```python
from build123d import *

# Parameters (mm, degrees)
ESQUISSE1_R        = 55
ESQUISSE1_R_2      = 1.227
ESQUISSE1_R_3      = 5
BOSS_EXTRU_1_DEPTH = 5
CONG_1_R           = 3
CHANFREIN1_SIZE    = 1


with BuildPart() as part:
    # Esquisse1 → Boss.-Extru.1 (new body)
    with BuildSketch(Plane.XY):
        Circle(ESQUISSE1_R)
        with Locations((-41.13620668, 23.75)):
            Circle(ESQUISSE1_R_2, mode=Mode.SUBTRACT)
        with Locations((-41.13620668, -23.75)):
            Circle(ESQUISSE1_R_2, mode=Mode.SUBTRACT)
        with Locations((0, -47.5)):
            Circle(ESQUISSE1_R_2, mode=Mode.SUBTRACT)
        with Locations((41.13620668, -23.75)):
            Circle(ESQUISSE1_R_2, mode=Mode.SUBTRACT)
        with Locations((41.13620668, 23.75)):
            Circle(ESQUISSE1_R_2, mode=Mode.SUBTRACT)
        with Locations((0, 47.5)):
            Circle(ESQUISSE1_R_2, mode=Mode.SUBTRACT)
        Circle(ESQUISSE1_R_3, mode=Mode.SUBTRACT)
        with BuildLine():
            ThreePointArc((36.043450899, -17.345594464), (34.641016151, 20), (3, 39.88734135))
            Line((3, 39.88734135), (3, 9.539392014))
            ThreePointArc((3, 9.539392014), (8.660254038, 5), (9.761355821, -2.171619796))
            Line((9.761355821, -2.171619796), (36.043450899, -17.345594464))
        make_face(mode=Mode.SUBTRACT)
        with BuildLine():
            ThreePointArc((-33.043450899, -22.541746887), (0, -40), (33.043450899, -22.541746887))
            Line((33.043450899, -22.541746887), (6.761355821, -7.367772218))
            ThreePointArc((6.761355821, -7.367772218), (0, -10), (-6.761355821, -7.367772218))
            Line((-6.761355821, -7.367772218), (-33.043450899, -22.541746887))
        make_face(mode=Mode.SUBTRACT)
        with BuildLine():
            Line((-3, 9.539392014), (-3, 39.88734135))
            ThreePointArc((-3, 39.88734135), (-34.641016151, 20), (-36.043450899, -17.345594464))
            Line((-36.043450899, -17.345594464), (-9.761355821, -2.171619796))
            ThreePointArc((-9.761355821, -2.171619796), (-8.660254038, 5), (-3, 9.539392014))
        make_face(mode=Mode.SUBTRACT)
    extrude(amount=BOSS_EXTRU_1_DEPTH)

    # Congé1
    cong_1_edges = [part.edges().sort_by_distance(p)[0] for p in [
        (-3, 39.88734135, 2.5),
        (-36.043450899, -17.345594464, 2.5),
        (-9.761355821, -2.171619796, 2.5),
        (-3, 9.539392014, 2.5),
        (33.043450899, -22.541746887, 2.5),
        (6.761355821, -7.367772218, 2.5),
        (-6.761355821, -7.367772218, 2.5),
        (-33.043450899, -22.541746887, 2.5),
        (3, 39.88734135, 2.5),
        (3, 9.539392014, 2.5),
        (9.761355821, -2.171619796, 2.5),
        (36.043450899, -17.345594464, 2.5),
    ]]
    fillet(cong_1_edges, radius=CONG_1_R)

    # Chanfrein1
    chanfrein1_edges = [part.edges().sort_by_distance(p)[0] for p in [
        (-5, 0, 5),
    ]]
    chamfer(chanfrein1_edges, length=CHANFREIN1_SIZE)


solid = part.part
```
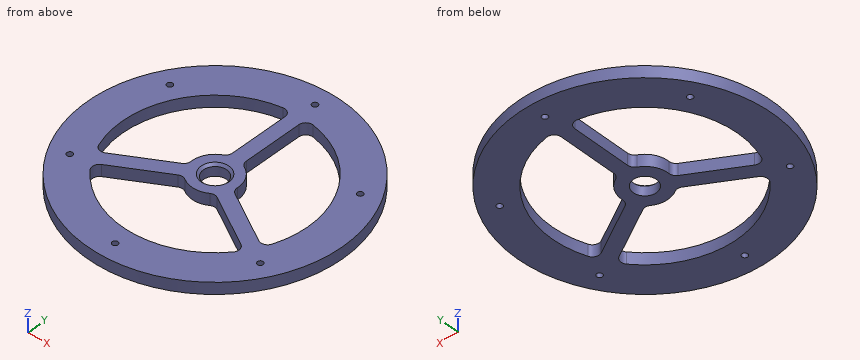
CAD build for the part. Positions are in the model's coordinates, mm. Round coordinates to 2 decimals unless told otherwise and drop trailing zeros. Order: outer loops, then holes, each group sorted by start corner. A loop starts at its lowest first (then second) coordinate and runs counter-clockwise, first axis right, second up. Notation, with made-up numbers: (-28, 85.5) -> (-6, 85.5) arc R9 cw to (-6, 94.5) -> close; hole circle Ø4 at (-19, -17.5). An arc over 180 degrees is marked (long way). One line per question, with ' | ' between items.
Q1. Drop flat-ended pins along their axis: pin 1 (2 mm diameter, centred on x = 1.5, z = 1.5, fed in from -Y); pin 2 (3 mm diameter, centred on x = -31, z = 3.5, fed in from -Y); pin 3 (1 mm diameter, centred on x = 6, z = 3.5, fed in from -Y). Give the stop position or say it passes through.
Completed:
pin 1: stops at y = -55 | pin 2: stops at y = -46.42 | pin 3: stops at y = -54.72
Q2. Slice it at A-A (x = -16). Write the cut outline in (y, z), then the cut area to 3 significant figures.
Completed:
outline: (-52.62, 0) -> (-36.66, 0) -> (-36.66, 5) -> (-52.62, 5) -> close; (-12.7, 0) -> (-5.77, 0) -> (-5.77, 5) -> (-12.7, 5) -> close; (36.66, 0) -> (52.62, 0) -> (52.62, 5) -> (36.66, 5) -> close | area: 194 mm^2
Q3. Slice it at C-C (z = 3.05). Give the number of separate pieces and of enclosed holes in the cut face, then the cut area to 3 significant figures.
Completed:
separate pieces: 1 | enclosed holes: 10 | area: 5,250 mm^2
Q4. Slice it at B-B (y = -30). Write the cut outline in (x, z).
Completed:
outline: (-46.1, 0) -> (-26.46, 0) -> (-26.46, 5) -> (-46.1, 5) -> close; (26.46, 0) -> (46.1, 0) -> (46.1, 5) -> (26.46, 5) -> close
Q5. Slice it at D-D (x = 19.5). Write the cut outline in (y, z), then the cut area to 3 significant figures.
Completed:
outline: (-51.43, 0) -> (-34.92, 0) -> (-34.92, 5) -> (-51.43, 5) -> close; (-14.72, 0) -> (-7.79, 0) -> (-7.79, 5) -> (-14.72, 5) -> close; (34.92, 0) -> (51.43, 0) -> (51.43, 5) -> (34.92, 5) -> close | area: 200 mm^2
Q6. Probe probe 1 along Y at (x, z) = (0, 2.55); probe 2 along X at (y, z) = (13.5, 3.15); probe 3 along Y at (x, z) = (-7, 1). List the from-to ranges inside material, lowest first.
Completed:
probe 1: y = -55 to -48.73, -46.27 to -40, -10 to -5, 5 to 46.27, 48.73 to 55 | probe 2: x = -53.32 to -37.65, -3 to 3, 37.65 to 53.32 | probe 3: y = -54.55 to -39.38, -7.96 to 7.14, 39.38 to 54.55
